```python
from build123d import *

# Parameters (mm, degrees)
SKETCH_1_W                = 55
SKETCH_1_H                = 42
EXTRUDE_1_DEPTH           = 20
SKETCH_2_W                = 6.5
SKETCH_2_H                = 9
CUT_EXTRUDE_1_DEPTH       = 68.203050526
SKETCH_3_W                = 6.5
SKETCH_3_H                = 30
CUT_EXTRUDE_2_DEPTH       = 68.203050526
SKETCH_4_W                = 6.5
SKETCH_4_H                = 30
CUT_EXTRUDE_3_DEPTH       = 68.203050526
SKETCH_5_W                = 6.5
SKETCH_5_H                = 9
CUT_EXTRUDE_4_DEPTH       = 68.203050526
SKETCH_6_W                = 3
SKETCH_6_H                = 5
HOLE_WIZARD_2_0_2_1_D     = 2
HOLE_WIZARD_2_0_2_1_DEPTH = 33
CUT_EXTRUDE_START         = -5
SKETCH_9_R                = 3
SKETCH_9_R_2              = 1.5
CUT_EXTRUDE_5_DEPTH       = 5
SKETCH_10_R               = 2
CUT_EXTRUDE_6_DEPTH       = 5


with BuildPart() as part:
    # 草图1 → 凸台-拉伸1 (new body)
    with BuildSketch(Plane.XY.offset(20)):
        with Locations((21, 21)):
            Rectangle(SKETCH_1_W, SKETCH_1_H)
    extrude(amount=-EXTRUDE_1_DEPTH)

    # 草图2 → 切除-拉伸1 (cut, through all)
    with BuildSketch(Plane(origin=(0, 0, 0), x_dir=(-1, 0, 0), z_dir=(0, 0, -1))):
        with Locations((3.25, 37.5)):
            Rectangle(SKETCH_2_W, SKETCH_2_H)
    extrude(amount=-CUT_EXTRUDE_1_DEPTH, mode=Mode.SUBTRACT)

    # 草图3 → 切除-拉伸2 (cut, through all)
    with BuildSketch(Plane(origin=(0, 0, 0), x_dir=(-1, 0, 0), z_dir=(0, 0, -1))):
        with Locations((3.25, 15)):
            Rectangle(SKETCH_3_W, SKETCH_3_H)
    extrude(amount=-CUT_EXTRUDE_2_DEPTH, mode=Mode.SUBTRACT)

    # 草图4 → 切除-拉伸3 (cut, through all)
    with BuildSketch(Plane(origin=(0, 0, 0), x_dir=(-1, 0, 0), z_dir=(0, 0, -1))):
        with Locations((-45.25, 15)):
            Rectangle(SKETCH_4_W, SKETCH_4_H)
    extrude(amount=-CUT_EXTRUDE_3_DEPTH, mode=Mode.SUBTRACT)

    # 草图5 → 切除-拉伸4 (cut, through all)
    with BuildSketch(Plane(origin=(0, 0, 0), x_dir=(-1, 0, 0), z_dir=(0, 0, -1))):
        with Locations((-45.25, 37.5)):
            Rectangle(SKETCH_5_W, SKETCH_5_H)
    extrude(amount=-CUT_EXTRUDE_4_DEPTH, mode=Mode.SUBTRACT)

    # 草图6 → 旋转1 (revolve)
    with BuildSketch(Plane(origin=(0, 0, 10.000000949), x_dir=(-1, 0, 0), z_dir=(0, 0, -1)), mode=Mode.PRIVATE) as revolve_1_sk:
        with Locations((-12, 44.5)):
            Rectangle(SKETCH_6_W, SKETCH_6_H)
    revolve(revolve_1_sk.sketch.rotate(Axis((10.5, 42, 10.000000949), (0, 1, 0)), 270), axis=Axis((10.5, 42, 10.000000949), (0, 1, 0)))

    # Ø2.0 (2) 直径孔1
    with Locations(Plane(origin=(0, 33, 0), x_dir=(1, 0, 0), z_dir=(0, 1, 0))):
        with Locations((46, -15.000000809), (-4, -5.000000809), (-4, -15.000000809), (46, -5.000000809)):
            Hole(HOLE_WIZARD_2_0_2_1_D / 2, depth=HOLE_WIZARD_2_0_2_1_DEPTH)

    # 草图9 → 切除-拉伸5 (cut)
    with BuildSketch(Plane(origin=(0, 47, 0), x_dir=(1, 0, 0), z_dir=(0, 1, 0)).offset(CUT_EXTRUDE_START)):
        with Locations((10.5, -10.000000949)):
            Circle(SKETCH_9_R)
        with Locations(Location((10.5, -10.000000949, 0), (0, 0, 270))):
            Circle(SKETCH_9_R_2, mode=Mode.SUBTRACT)
    extrude(amount=CUT_EXTRUDE_5_DEPTH, mode=Mode.SUBTRACT)

    # 草图10 → 切除-拉伸6 (cut)
    with BuildSketch(Plane(origin=(0, 33, 0), x_dir=(1, 0, 0), z_dir=(0, 1, 0))):
        with Locations(Location((46, -15.000000809, 0), (0, 0, 270))):
            Circle(SKETCH_10_R)
        with Locations(Location((46, -5.000000809, 0), (0, 0, 270))):
            Circle(SKETCH_10_R)
        with Locations(Location((-4, -5.000000809, 0), (0, 0, 270))):
            Circle(SKETCH_10_R)
        with Locations(Location((-4, -15.000000809, 0), (0, 0, 270))):
            Circle(SKETCH_10_R)
    extrude(amount=-CUT_EXTRUDE_6_DEPTH, mode=Mode.SUBTRACT)


solid = part.part
```
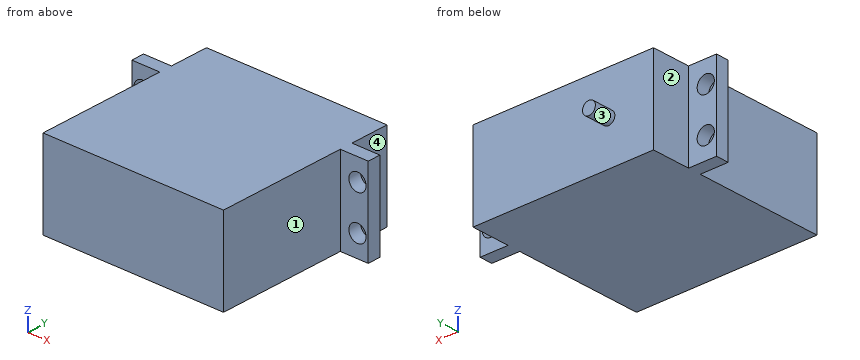
Model file for the job. Use its own axes, mm. Face numbers are marked on the shaded views. A direction names the side the tool comes from. Give positions to 0.01 mm unless a question says otherwise; leave off trailing zeros. Write each loop counter-clockwise with the first axis right and the second up, starting at its lowest first coordinate (ties: lowest second). Pieces come first, ordered by that corner, then holes. Notation, with made-up numbers: M 47.5,1.5 L 77.5,1.5 A21 ccw 77.5,11.5 Z; hole C 19.5,-20.5 d7. An arc over 180 degrees is marked long. Use a Markdown table: item, result.
1) Cut at C-C (z = 10). List the corners of the cut face in (x, y).
Responses:
| item | result |
|---|---|
| outline | M -6.5,30 L 0,30 L 0,0 L 42,0 L 42,30 L 48.5,30 L 48.5,33 L 42,33 L 42,42 L 12,42 L 12,47 L 9,47 L 9,42 L 0,42 L 0,33 L -6.5,33 Z |
2) Cut at D-D (x = 10.5). List the corners of the cut face in (y, z).
Responses:
| item | result |
|---|---|
| outline | M 0,0 L 42,0 L 42,8.5 L 47,8.5 L 47,11.5 L 42,11.5 L 42,20 L 0,20 Z |
3) Drill centre lines: line 1 (X direction, y = 31.2, z = 5); line 2 (Y direction, x = 14, z = 14). Where is each one in solid material? Low to high. Write a range as from..to.
Responses:
| item | result |
|---|---|
| line 1 | x = -6.5..-6, -2..44, 48..48.5 |
| line 2 | y = 0..42 |
4) Cut at A-A (x = -4). List the corners of the cut face in (y, z).
Responses:
| item | result |
|---|---|
| outline | M 30,0 L 33,0 L 33,3 L 30,3 Z; M 30,7 L 33,7 L 33,13 L 30,13 Z; M 30,17 L 33,17 L 33,20 L 30,20 Z |
5) Pin check, flat tips, straight feed: pin 1 (10 mm diameter, centred on x = 32, y = 6.5, fed in from -Z); pin 2 (10 mm diameter, centred on y = 18, z = 12, fed in from +X); pin 3 (1.5 mm diameter, centred on x = 8, z = 2.5, fed in from +Y); pin 4 (5 mm diameter, centred on x = -4, z = 5, fed in from -Y). Stop position of each tip, or through.
Responses:
| item | result |
|---|---|
| pin 1 | stops at z = 0 |
| pin 2 | stops at x = 42 |
| pin 3 | stops at y = 42 |
| pin 4 | stops at y = 30 |
6) Tool access for the marked faces 1, 2, 3 and 4: list every direction of +Z, -Z, +X, -X, +Y, -Y with a clear straight run to the whole face (end or side of a thin tool).
Responses:
| item | result |
|---|---|
| face 1 | +Z, -Z, +X, -Y |
| face 2 | +Z, -Z, -X, +Y |
| face 3 | +Y |
| face 4 | +Z, -Z, +X, +Y |
7) Cut at B-B (z = 15). List the corners of the cut face in (x, y).
Responses:
| item | result |
|---|---|
| outline | M -6.5,30 L -6,30 L -6,33 L -6.5,33 Z; M -2,30 L 0,30 L 0,0 L 42,0 L 42,30 L 44,30 L 44,33 L 42,33 L 42,42 L 0,42 L 0,33 L -2,33 Z; M 48,30 L 48.5,30 L 48.5,33 L 48,33 Z |
